from build123d import *

# Parameters (mm, degrees)
F1_DEPTH = 25
F2_R     = 4
F3_DEPTH = 22.001
F4_R     = 5


with BuildPart() as f1:
    # F0 (on Top) → F1 (new body)
    with BuildSketch(Plane.XY):
        Polygon((5, 47.435442), (-17, 47.435442), (-17, -2.564558), (-22.601457, -16.47943), (-9.883268, -24.432269), (5, -22.564558), align=None)
    extrude(amount=F1_DEPTH)

    # F2 (on face) → F3 (cut, through all)
    with BuildSketch(Plane(origin=(-17, 0, 0), x_dir=(0, -1, 0), z_dir=(-1, 0, 0))):
        with Locations((-33.117216, 15)):
            Circle(F2_R)
    extrude(amount=-F3_DEPTH, mode=Mode.SUBTRACT)

    # F4
    f4_edges = [f1.edges().sort_by_distance(p)[0] for p in [
        (-6, 47.435442, 25),
        (-17, 22.435442, 25),
        (-19.800729, -9.521994, 25),
        (-16.242363, -20.45585, 25),
        (-2.441634, -23.498413, 25),
        (5, 12.435442, 25),
    ]]
    fillet(f4_edges, radius=F4_R)


solid = f1.part
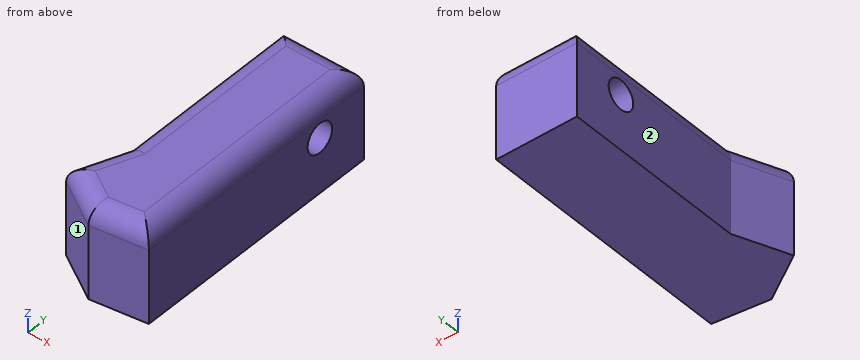
For this review, take the finished solid that the model builds, in its own axes (mm). Face numbers are marked on the shaded views. A direction names the side the tool comes from. Round coordinates to 2 decimals unless told otherwise and drop trailing zeros. Loops run counter-clockwise (first coordinate to the right, second up) from the corner with the lowest first, then second, coordinate; pieces in that order, holes last. Notation, with made-up numbers: (52, 38.25) - (97, 38.25) arc R9 cw to (97, 52.25) - close; hole circle Ø5 at (-28, 7.5). An arc over 180 degrees is marked (long way). Put each result on its own line as item: value. Start each with the question number.
1. Consider section B-B on y = 31. State the section outline as (x, z) points.
2. For probe 1 along X at (y, z) = (1, 20.25); probe 2 along Y at (x, z) = (-4.5, 18.25); probe 3 along Y at (x, z) = (3.75, 15.25), list the stretches that pass through material, from the lowest coordinate up. Write a range as [from, to].
3. Insertion check: P1, Ø1.5, axis at x = -8, z = 13.5, coming from the -Y side; P2, Ø5, axis at y = 9.5, z = 10, coming from the -X side; P3, Ø1, axis at x = -9, z = 6.5, coming from the -Y side. Each pin has a flat end and moves straight along its axis. Give the tip position at first contact, or say it passes through.
4. Consider section C-C on z = 7.75. State the section outline as (x, y) points, plus the area to 3 significant figures.
5. Consider section A-A on z = 15. State the section outline as (x, y) points, plus the area to 3 significant figures.
6. Consider section D-D on y = 3. State the section outline as (x, z) points, plus the area to 3 significant figures.
7. For the marked faces 1 and 2, list the 3-axis set-ups (+Z, -Z, +X, -X, +Y, -Y) from which the entire face can be reached by the end or side of a thin tool; tool diameter is ignored.
Result sheet:
1. outline: (-17, 0) - (5, 0) - (5, 11.61) - (-17, 11.61) - close; (-17, 18.39) - (5, 18.39) - (5, 20) arc R5 ccw to (0, 25) - (-12, 25) arc R5 ccw to (-17, 20) - close
2. probe 1: [-16.99, 4.99]
2. probe 2: [-23.76, 30.79], [35.45, 47.44]
2. probe 3: [-22.72, 29.13], [37.11, 47.44]
3. P1: y = -24.29
3. P2: x = -17
3. P3: y = -24.38
4. outline: (-22.6, -16.48) - (-9.88, -24.43) - (5, -22.56) - (5, 47.44) - (-17, 47.44) - (-17, -2.56) - close
4. area: 1,600 mm^2
5. outline: (-22.6, -16.48) - (-9.88, -24.43) - (5, -22.56) - (5, 29.12) - (-17, 29.12) - (-17, -2.56) - close; (-17, 37.12) - (5, 37.12) - (5, 47.44) - (-17, 47.44) - close
5. area: 1,420 mm^2
6. outline: (-17, 0) - (5, 0) - (5, 20) arc R5 ccw to (0, 25) - (-12, 25) arc R5 ccw to (-17, 20) - close
6. area: 539 mm^2
7. face 1: +Z, -Z, -X, -Y
7. face 2: +Z, -Z, -X, +Y
